The listing builds one solid part. Answer for the finished solid, in the listing's coordinates (mm). Face numbers are marked on the shaded views. A direction names the side the tool comes from. Coordinates: 2 decimals unless noted, no trailing zeros. Order: outer loops, then holes, each group sorted by start corner. A loop starts at its lowest first (then second) coordinate and runs counter-clockwise, first axis right, second up. Notation, with made-up numbers: M 71.25,75.5 L 86.25,75.5 A31 ccw 86.25,104.5 Z; hole C 85.5,22.25 d3. An arc over 180 degrees is marked long. One line per item, written item: value. Start each with the question number.
Q1. The part is cut by section C-C on y = 0. Give the vertices of the cut face in (x, z).
Q2. Straight lines are drawn through the part: line 1 along Y through (x, z) = (4.25, 18.5); line 2 along Y through (x, z) = (2, 3.25); line 3 along Y through (x, z) = (2.25, 19.25). For each, find the intervals that lie inside material, in ascending order. Write a range as [from, to].
Q3. Determine the mould class of the marked faces 1, 2 and 3 for opening direction Y: pulls with the +Y half, pulls with the -Y half, needs draft (parallel to the pull), parting line crosses it, or undercut.
Q4. Each of these flat-tipped pins is pushed along its axis until it touches: pin 1 Ø6.5 at (x, z) = (0.5, 12) entering from +Y; pin 2 Ø1.5 at (y, z) = (5.5, 3) entering from -X; pin 3 Ø8 at (y, z) = (2.5, 16) entering from -X; pin 4 Ø4 at (x, z) = (-2.5, 5) entering from -Y. Where does it stop, or does it pass through?
Q5. The part is cut by section D-D on z = 3.25. Give the vertices of the cut face in (x, y), then the cut area to 3 significant figures.
Q6. The part is cut by section A-A on z = 14.25. Give the vertices of the cut face in (x, y), then the cut area to 3 significant figures.
Q7. For the marked faces 4 and 5, determine the directions among +Z, -Z, +X, -X, +Y, -Y from which every point of the face is accessible in a straight line to the end or side of a thin tool.
Q8. The part is cut by section B-B on x = 0. Give the vertices of the cut face in (y, z), then the cut area to 3 significant figures.
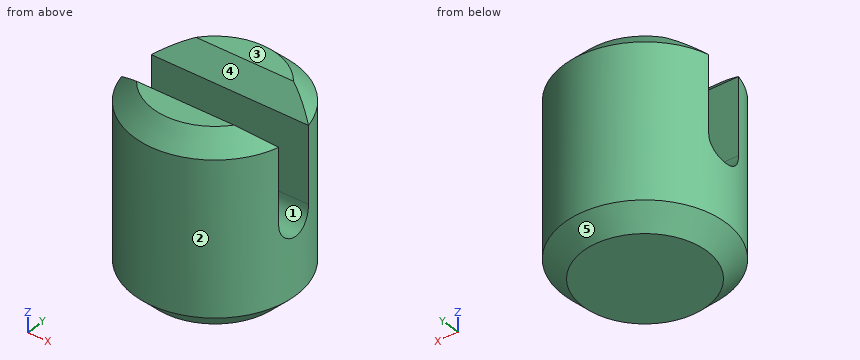
```python
from build123d import *

# Parameters (mm, degrees)
BOX_W                   = 20
BOX_H                   = 4
BOX_DEPTH               = 10
CYLINDER001_R           = 2
CYLINDER001_DEPTH       = 20
CYLINDER001_PITCH_ANGLE = 90
CYLINDER_R              = 8.5
CYLINDER_DEPTH          = 20
CHAMFER_SIZE            = 2


with BuildPart() as cube:
    # Box → Box (new body)
    with BuildSketch(Plane(origin=(-10, -2, 10), x_dir=(1, 0, 0), z_dir=(0, 0, 1))):
        with Locations((10, 2)):
            Rectangle(BOX_W, BOX_H)
    extrude(amount=BOX_DEPTH)


with BuildPart() as fusion:
    # Cylinder001 → Cylinder001 (new body)
    with BuildSketch(Plane.XY):
        Circle(CYLINDER001_R)
    extrude(amount=CYLINDER001_DEPTH)


with BuildPart() as fusion_1:
    # Cylinder001 pitch: moved
    add(fusion.part.rotate(Axis((0, 0, 0), (0, 1, 0)), CYLINDER001_PITCH_ANGLE))


with BuildPart() as fusion_2:
    # Cylinder001 placement: moved
    add(fusion_1.part.moved(Location((-10, 0, 10))))

    # Fusion: union Cube
    add(cube.part)


with BuildPart() as chamfer_body:
    # Cylinder → Cylinder (new body)
    with BuildSketch(Plane.XY):
        Circle(CYLINDER_R)
    extrude(amount=CYLINDER_DEPTH)

    # Cut: cut Fusion
    add(fusion_2.part, mode=Mode.SUBTRACT)

    # Chamfer
    chamfer_edges = [chamfer_body.edges().sort_by_distance(p)[0] for p in [
        (0, 8.5, 20),
        (0, -8.5, 20),
        (-8.5, 0, 0),
        (0, 2, 20),
        (0, -2, 20),
    ]]
    chamfer(chamfer_edges, length=CHAMFER_SIZE)


solid = chamfer_body.part
```
Output:
1. outline: M -8.5,2 L -6.5,0 L 6.5,0 L 8.5,2 L 8.5,8 L -8.5,8 Z
2. line 1: y = [-6.78, -2.5], [2.5, 6.78]
2. line 2: y = [-8.26, 8.26]
2. line 3: y = [-6.89, -3.25], [3.25, 6.89]
3. face 1: undercut
3. face 2: parting line crosses it
3. face 3: needs draft
4. pin 1: stops at y = 8.5
4. pin 2: stops at x = -7.05
4. pin 3: stops at x = -8.26
4. pin 4: stops at y = -8.49
5. outline: C 0,0 d17
5. area: 227 mm^2
6. outline: M -8.26,-2 A8.5 ccw 8.26,-2 Z; M -8.26,2 L 8.26,2 A8.5 ccw Z
6. area: 160 mm^2
7. face 4: +Z, +X, -X
7. face 5: -Z
8. outline: M -8.5,2 L -6.5,0 L 6.5,0 L 8.5,2 L 8.5,18 L 6.5,20 L 4,20 L 2,18 L 2,10 A2 cw -2,10 L -2,18 L -4,20 L -6.5,20 L -8.5,18 Z
8. area: 282 mm^2
